Part model, mm, in its own coordinate system. A direction names the side the tool comes from. Round coordinates to 2 decimals unless told otherwise and drop trailing zeros. Order: outer loops, then holes, each group sorted by start corner. A loop starts at its lowest first (then second) coordinate and runs counter-clockwise, first axis right, second up. Notation, with made-up numbers: (0, 56.25) - (51, 56.25) arc R12 cw to (51, 68.25) - close; hole circle Ø3 at (35, 78). An arc over 180 degrees is marked (long way). Return JSON: item names as keys, results as strings. Group by question number.
Item 1: Probe probe 1 along Y at (x, z) = (15.5, 45.5); probe 2 along X at (y, z) = (-123.5, 6); probe 3 along Y at (x, z) = (22, 57). List the from-to ranges inside material, lowest first.
Item 2: Saw through at D-D on x = 16.5. State how many separate pieces and enclosed holes the cut face has, and give its area (3 significant figures).
Item 3: Tool access for faces 5 (the face through (54, -75, 25.4)), 6 (the face through (0, -75, 32)): list every direction of +Z, -Z, +X, -X, +Y, -Y with a clear straight run to the whole face (end or side of a thin tool).
Item 4: Saw through at C-C on z = 9. List the corners of the cut face in (x, y) (3 decimals).
Item 5: Saw through at B-B on x = 51.5. List the corners of the cut face in (y, z).
Item 6: Drop a flat-ended pin along its axis: pin 1 (6 mm diameter, centred on x = 54, y = -81.5, fed in from +Z). Give the stop position or say it passes through.
Item 7: Two-plate mould, pull along Y, no slides. Class faces 1 (the face through (34, -75, 0)), 2 (the face through (16.652, -20.643, 32.18)), 3 (the face through (16.652, -115.893, 32.18)), 4 (the face through (27, -152.4, 25)): released by +Y, released by -Y, zero draft, split by the parting line, or undercut.
Item 8: Saw through at A-A on y = -76.2. List the corners of the cut face in (x, z).
```python
from build123d import *

# Parameters (mm, degrees)
F1_DEPTH = 152.4
F2_R     = 7.99973
F3_DEPTH = 63.501
F4_SIZE  = 1.016


with BuildPart() as f1:
    # F0 (on Front) → F1 (new body)
    with BuildSketch(Plane.XZ):
        Polygon((0, 63.5), (0, 0), (69.85, 0), (69.85, 25.4), (38.1, 25.4), (38.1, 63.5), align=None)
    extrude(amount=F1_DEPTH)

    # F2 (on face) → F3 (cut, through all)
    with BuildSketch(Plane.XY.offset(63.5)):
        with Locations((17.6930073649, -28.575)):
            Circle(F2_R)
        with Locations((17.6930073649, -76.2)):
            Circle(F2_R)
        with Locations((17.6930073649, -123.825)):
            Circle(F2_R)
    extrude(amount=-F3_DEPTH, mode=Mode.SUBTRACT)

    # F4
    f4_edges = [f1.edges().sort_by_distance(p)[0] for p in [
        (0, -152.4, 31.75),
        (34.925, -152.4, 0),
        (69.85, -152.4, 12.7),
        (53.975, -152.4, 25.4),
        (38.1, -152.4, 44.45),
        (19.05, -152.4, 63.5),
        (0, 0, 31.75),
        (34.925, 0, 0),
        (69.85, 0, 12.7),
        (53.975, 0, 25.4),
        (38.1, 0, 44.45),
        (19.05, 0, 63.5),
        (38.1, -76.2, 63.5),
        (0, -76.2, 63.5),
        (9.693277, -123.825, 63.5),
        (9.693277, -76.2, 63.5),
        (9.693277, -28.575, 63.5),
        (69.85, -76.2, 0),
        (69.85, -76.2, 25.4),
        (0, -76.2, 0),
        (9.693277, -123.825, 0),
        (9.693277, -76.2, 0),
        (9.693277, -28.575, 0),
    ]]
    chamfer(f4_edges, length=F4_SIZE)


solid = f1.part
```
Filled in:
{
 "1": {"probe 1": "y = -152.4 to -131.52, -116.13 to -83.89, -68.51 to -36.27, -20.88 to 0", "probe 2": "x = 0 to 9.7, 25.69 to 69.85", "probe 3": "y = -152.4 to -130.57, -117.08 to -82.94, -69.46 to -35.32, -21.83 to 0"},
 "2": {"separate pieces": "4", "enclosed holes": "0", "area": "6,660 mm^2"},
 "3": {"face 5": "+Z, +X, +Y, -Y", "face 6": "+Z, -Z, -X, +Y, -Y"},
 "4": {"outline": "(0, -151.384) - (1.016, -152.4) - (68.834, -152.4) - (69.85, -151.384) - (69.85, -1.016) - (68.834, 0) - (1.016, 0) - (0, -1.016) - close; hole circle Ø15.999 at (17.693, -123.825); hole circle Ø15.999 at (17.693, -76.2); hole circle Ø15.999 at (17.693, -28.575)"},
 "5": {"outline": "(-152.4, 1.02) - (-151.38, 0) - (-1.02, 0) - (0, 1.02) - (0, 24.38) - (-1.02, 25.4) - (-151.38, 25.4) - (-152.4, 24.38) - close"},
 "6": {"pin 1": "stops at z = 25.4"},
 "7": {"face 1": "zero draft", "face 2": "undercut", "face 3": "undercut", "face 4": "released by -Y"},
 "8": {"outline": "(0, 1.02) - (1.02, 0) - (8.68, 0) - (9.69, 1.02) - (9.69, 62.48) - (8.68, 63.5) - (1.02, 63.5) - (0, 62.48) - close; (25.69, 1.02) - (26.71, 0) - (68.83, 0) - (69.85, 1.02) - (69.85, 24.38) - (68.83, 25.4) - (38.1, 25.4) - (38.1, 62.48) - (37.08, 63.5) - (26.71, 63.5) - (25.69, 62.48) - close"}
}
